```python
from build123d import *

# Parameters (mm, degrees)
BOSS_EXTRUDE3_DEPTH  = 74
SKETCH5_R            = 5
CUT_EXTRUDE1_DEPTH   = 91.144328718
M3_CLEARANCE_HOLE2_D = 3.4
SKETCH11_R           = 1.5
CUT_EXTRUDE2_DEPTH   = 90.162772501
FILLET1_R            = 20


with BuildPart() as part:
    # Sketch4 → Boss-Extrude3 (new body)
    with BuildSketch(Plane.XY):
        Polygon((0, 0), (25, 0), (25, 45), (23, 45), (23, 2), (0, 2), align=None)
    extrude(amount=BOSS_EXTRUDE3_DEPTH)

    # Sketch5 → Cut-Extrude1 (cut, through all)
    with BuildSketch(Plane(origin=(25, 0, 0), x_dir=(0, 0, -1), z_dir=(1, 0, 0))):
        with Locations((-37, 30.5)):
            Circle(SKETCH5_R)
    extrude(amount=-CUT_EXTRUDE1_DEPTH, mode=Mode.SUBTRACT)

    # M3 Clearance Hole2 (through all)
    with Locations(Plane(origin=(25, 0, 0), x_dir=(0, 0, -1), z_dir=(1, 0, 0))):
        with Locations((-30.75, 14.174682453), (-30.75, 35.825317547), (-49.5, 25)):
            Hole(M3_CLEARANCE_HOLE2_D / 2)

    # Sketch11 → Cut-Extrude2 (cut, through all)
    with BuildSketch(Plane(origin=(0, 2, 0), x_dir=(1, 0, 0), z_dir=(0, 1, 0))):
        with Locations(Location((7, -67, 0), (0, 0, 270))):
            Circle(SKETCH11_R)
        with Locations(Location((18, -67, 0), (0, 0, 270))):
            Circle(SKETCH11_R)
        with Locations(Location((18, -7, 0), (0, 0, 90))):
            Circle(SKETCH11_R)
        with Locations(Location((7, -7, 0), (0, 0, 90))):
            Circle(SKETCH11_R)
    extrude(amount=-CUT_EXTRUDE2_DEPTH, mode=Mode.SUBTRACT)

    # Fillet1
    fillet1_edges = [part.edges().sort_by_distance(p)[0] for p in [
        (24, 45, 74),
        (24, 45, 0),
    ]]
    fillet(fillet1_edges, radius=FILLET1_R)


solid = part.part
```
Check sheet for the modelled part. Datum: model origin and axes. Units: mm. A direction names the side the tool comes from. Round coordinates to 2 decimals unless told otherwise and drop trailing zeros. Loops run counter-clockwise (first coordinate to the right, second up) from the corner with the lowest first, then second, coordinate; pieces in that order, holes last. Notation, with made-up numbers: (-13, 65.5) - (46, 65.5) arc R17 cw to (46, 83.5) - close; hole circle Ø3 at (89.5, 21). An arc over 180 degrees is marked (long way). Answer as a JSON object with one key per item and string values. Group by question number.
Q1. Scan lines: line 1 along Y through (x, z) = (24.1, 30.75); line 2 along Y through (x, z) = (23.65, 49.5); line 3 along Y through (x, z) = (14.5, 32). Record each from-to range of solid material in increasing order. Write a range as [from, to].
Q2. Gauge pin test, flat ends, axial feed: P1, Ø4, axis at y = 35.83, z = 30.75, coming from the +X side; P2, Ø2, axis at y = 25, z = 49.5, coming from the +X side; P3, Ø1.5, axis at x = 15, z = 60.5, coming from the +Y side. Record the tip position at first contact, or that the pin passes through.
Q3. Sectioned sample at D-D, the plane y = 30.5. Enter the section's corners in (x, z), plus the area to 3 significant figures.
Q4. Mould release check, pull along Y, two halves, no side actions. Record for faces 1 (the face through (12, 0, 36)), 2 (the face through (23, 24, 36)), 3 (the face through (23.99, 36.34, 32.37)): released by +Y, released by -Y, zero draft, split by the parting line, or undercut.
Q5. Set-up check for faces 4 (the face through (12, 2, 36)), 5 (the face through (18, 1, 0)): record each of +Z, -Z, +X, -X, +Y, -Y from which the full face is reachable in a straight line by a thin tool's end or side.
Q6. Sectioned sample at B-B, the plane x = 7. Enter the section's corners in (y, z), plus the area to 3 significant figures.
Q7. Sectioned sample at C-C, the plane z = 49.5. Enter the section's corners in (x, y).
Q8. Sectioned sample at A-A, the plane z = 30.75. Enter the section's corners in (x, y).
Solution:
{
 "1": {"line 1": "y = [0, 12.47], [15.87, 34.13], [37.53, 45]", "line 2": "y = [0, 23.3], [26.7, 45]", "line 3": "y = [0, 2]"},
 "2": {"P1": "stops at x = 25", "P2": "passes through", "P3": "stops at y = 2"},
 "3": {"outline": "(23, 0.77) - (25, 0.77) - (25, 32) - (23, 32) - close; (23, 42) - (25, 42) - (25, 73.23) - (23, 73.23) - close", "area": "125 mm²"},
 "4": {"face 1": "released by -Y", "face 2": "zero draft", "face 3": "undercut"},
 "5": {"face 4": "+Z, -Z, -X, +Y", "face 5": "-Z, +X, -X, +Y, -Y"},
 "6": {"outline": "(0, 0) - (2, 0) - (2, 5.5) - (0, 5.5) - close; (0, 8.5) - (2, 8.5) - (2, 65.5) - (0, 65.5) - close; (0, 68.5) - (2, 68.5) - (2, 74) - (0, 74) - close", "area": "136 mm²"},
 "7": {"outline": "(0, 0) - (25, 0) - (25, 23.3) - (23, 23.3) - (23, 2) - (0, 2) - close; (23, 26.7) - (25, 26.7) - (25, 45) - (23, 45) - close"},
 "8": {"outline": "(0, 0) - (25, 0) - (25, 12.47) - (23, 12.47) - (23, 2) - (0, 2) - close; (23, 15.87) - (25, 15.87) - (25, 34.13) - (23, 34.13) - close; (23, 37.53) - (25, 37.53) - (25, 45) - (23, 45) - close"}
}
